Autodesk Inventor part; units mm, degrees
ref_plane "YZ Plane" through (0, 0, 0) normal (1, 0, 0) x (0, 1, 0)
ref_plane "XZ Plane" through (0, 0, 0) normal (0, 1, 0) x (-1, 0, 0)
ref_plane "XY Plane" through (0, 0, 0) normal (0, 0, 1) x (1, 0, 0)
sketch "Sketch1" plane through (0, 0, 0) normal (0, 0, 1) x (1, 0, 0)
  line L0 (0, 0) -> (-10.4993, 120.0076)
  line L1 (-10.4993, 120.0076) -> (113.201, -41.2018)
  line L2 (113.201, -41.2018) -> (0, 0)
  dimension "d23" = 115
  dimension "d24" = 203.2
  dimension "d31" = 32.5
extrude "Extrusion1" add sketch "Sketch1" along normal mid plane 19.05
sketch "Sketch2" plane through (0, 0, 0) normal (0, 0, 1) x (1, 0, 0)
  line L0 (8.9599, 6.8752) -> (1.8376, 88.2833)
  line L1 (1.8376, 88.2833) -> (85.7507, -21.0744)
  line L2 (85.7507, -21.0744) -> (8.9599, 6.8752)
  line L3 (0, 0) -> (-10.4993, 120.0076)
  line L4 (-10.4993, 120.0076) -> (113.201, -41.2018)
  line L5 (113.201, -41.2018) -> (0, 0)
  dimension "d4" = 9.525
  dimension "d5" = 9.525
  dimension "d6" = 9.525
extrude "Extrusion2" cut sketch "Sketch2" against normal through all both and the other way through all contours L0 L1 L2
fillet "Fillet1" radius 3.175 3 edges at (-10.4993, 120.0076, 0) (0, 0, 0) (113.201, -41.2018, 0)
fillet "Fillet2" radius 3.175 3 edges at (1.8376, 88.2833, 0) (8.9599, 6.8752, 0) (85.7507, -21.0744, 0)
equation "\"d23\" = longAngle"
equation "\"d24\" = maxLength"
equation "\"d31\" = basicAngle"
equation "\"d2\" = width"
equation "\"d4\" = wallThickness"
equation "\"d5\" = wallThickness"
equation "\"d6\" = wallThickness"
equation "\"d32\" = fillet"
equation "\"d33\" = fillet"
equation "\"maxLength\" = 203.2"
equation "\"width\" = 19.05"
equation "\"wallThickness\" = 9.525"
equation "\"longAngle\" = 115deg"
equation "\"fillet\" = 3.175"
properties part number "stopForSaltChute"
For this review, take the finished solid that the model builds, in its own axes (mm). A direction names the side the tool comes from. Round coordinates to 2 decimals unless told otherwise and drop trailing zeros. Loops run counter-clockwise (first coordinate to the right, second up) from the corner with the lowest first, then second, coordinate; pieces in that order, holes last.
Q1. Machinability: for faces 5 (the face through (-4.797, 54.836, -0.133)), 6 (the face through (43.3, 34.25, 0.13)), which of the approach directions +Z, -Z, +X, -X, +Y, -Y give a long, thin tool a straight path to every point of the face, cutting with its end or side? Answer none if there is none.
Result sheet:
face 5: +Z, -Z, -X, -Y
face 6: +Z, -Z
Q2. Add section C-C on x = 28.5. Write out the cut boundary in (y, z) (3 decimals).
Result sheet:
outline: (-10.373, -9.525) - (-0.237, -9.525) - (-0.237, 9.525) - (-10.373, 9.525) - close; (53.536, -9.525) - (69.183, -9.525) - (69.183, 9.525) - (53.536, 9.525) - close
Q3. To check wall thickness, follow line 1 along X through (y, z) = (69.5, -5.75); line 2 along Y through (x, z) = (27, 4.25); line 3 along X through (y, z) = (23, 5). State the ranges of each line that lie inside material, in increasing order.
Result sheet:
line 1: x = -6.08 to 3.48, 16.25 to 28.26
line 2: y = -9.83 to 0.31, 55.49 to 71.14
line 3: x = -2.01 to 7.55, 51.93 to 63.94
Q4. Add section D-D on x = 86. Write out the cut boundary in (y, z) (3 decimals), plus the area to 3 significant figures.
Result sheet:
outline: (-31.301, -9.525) - (-5.753, -9.525) - (-5.753, 9.525) - (-31.301, 9.525) - close
area: 487 mm2
Q5. Mouldability with a two-part tool opening along X and no side actions: class faces 1 (the face through (-7.59, 112.37, -0.13)), 2 (the face through (5.827, 42.681, 0.133)), 3 (the face through (53.14, -19.34, -0.13)), 4 (the face through (79.127, -16.289, 0.133)) as +X half, -X half, draft (parallel to the pull), parting line (faces both ways), or undercut.
Result sheet:
face 1: parting line
face 2: undercut
face 3: -X half
face 4: undercut
Q6. Insertion check: pin 1 Ø4 at (y, z) = (35, 4.5) entering from -X; pin 2 Ø10 at (x, y) = (36.5, 70.5) entering from +Z; pin 3 Ø8 at (y, z) = (80.5, -1) entering from -X; pin 4 Ø4 at (y, z) = (51.5, 0) entering from -X. Each pin has a flat end and moves straight along its axis. Give the tip position at first contact, or say it passes through.
Result sheet:
pin 1: stops at x = -3.24
pin 2: passes through
pin 3: stops at x = -7.39
pin 4: stops at x = -4.68
Q7. Add section B-B on y = 51. Write out the cut boundary in (x, z) (3 decimals).
Result sheet:
outline: (-4.462, -9.525) - (5.099, -9.525) - (5.099, 9.525) - (-4.462, 9.525) - close; (30.446, -9.525) - (42.452, -9.525) - (42.452, 9.525) - (30.446, 9.525) - close
